Work out the finished part from the listing and answer in its coordinate system (mm). Coordinates: 2 decimals unless noted, no trailing zeros. Loops run counter-clockwise (first coordinate to the right, second up) from the corner with the lowest first, then second, coordinate; pieces in that order, holes last. Notation, with made-up numbers: (4.25, -13) - (43.25, -13) arc R32 ccw to (43.25, 16) - close; hole circle Ø10 at (76, -26.5). An arc over 180 degrees is marked (long way). Write each question's results on one line, items separated by ' | '. Start each with the question number.
1. Each of these flat-tipped pins is pushed along its axis until it touches: P1, Ø6.5, axis at x = 0, z = 127, coming from the +Y side; P2, Ø1.5, axis at x = 3, y = -9, coming from the -Z side. Where does it stop, or does it pass through?
2. Determine the mould class of faces 1 (the flat face through (-11, -10, 2)), 2 (the flat face through (0, -1.5, 2)), 3 (the cylindrical face through (-0.716, -10.152, -121.547)) for opening direction X: released by +X, released by -X, zero draft, split by the parting line, or undercut.
3. Find the intervals of material crossed by line 1 along Z through (x, y) = (0.75, -4.25); line 2 along Z through (x, y) = (-5, -12); line 3 along X through (y, z) = (-13.75, -45.5), in increasing order. Write a range as [from, to].
4. A cutting plane is placed at B-B on x = 2.75. Determine the outline of the cut face in (y, z).
5. A cutting plane is placed at A-A on y = -7. Determine the outline of the cut face in (x, z).
from build123d import *

# Parameters (mm, degrees)
F0_R     = 5.5
F1_DEPTH = 19.05
F2_DEPTH = 1.5


# Not quite as in the source:
# - a length typed as a fraction of an inch, garbled in the dataset ("3 / 203.2 mm" for 3/8 in), is restored
# - a feature names something its author has since deleted; it is built from what else it names


with BuildPart() as f1:
    # F0 (on Front) → F1 (new body)
    with BuildSketch(Plane.XZ):
        with BuildLine():
            Line((11, -127), (11, 127))
            ThreePointArc((11, 127), (7.7781745931, 134.7781745931), (0, 138))
            ThreePointArc((0, 138), (-7.7781745931, 134.7781745931), (-11, 127))
            Line((-11, 127), (-11, -127))
            ThreePointArc((-11, -127), (-7.7781745931, -134.7781745931), (0, -138))
            ThreePointArc((0, -138), (7.7781745931, -134.7781745931), (11, -127))
        make_face()
        with Locations((0, -127)):
            Circle(F0_R, mode=Mode.SUBTRACT)
        with Locations((0, -41.9999994338)):
            Circle(F0_R, mode=Mode.SUBTRACT)
        with Locations((0, 127)):
            Circle(F0_R, mode=Mode.SUBTRACT)
    extrude(amount=F1_DEPTH)

    # F0 (on Front) → F2 (cut)
    with BuildSketch(Plane.XZ):
        with BuildLine():
            Line((11, -127), (11, 127))
            ThreePointArc((11, 127), (7.7781745931, 134.7781745931), (0, 138))
            ThreePointArc((0, 138), (-7.7781745931, 134.7781745931), (-11, 127))
            Line((-11, 127), (-11, -127))
            ThreePointArc((-11, -127), (-7.7781745931, -134.7781745931), (0, -138))
            ThreePointArc((0, -138), (7.7781745931, -134.7781745931), (11, -127))
        make_face()
        with Locations((0, -127)):
            Circle(F0_R, mode=Mode.SUBTRACT)
        with Locations((0, -41.9999994338)):
            Circle(F0_R, mode=Mode.SUBTRACT)
        with Locations((0, 127)):
            Circle(F0_R, mode=Mode.SUBTRACT)
    extrude(amount=F2_DEPTH, mode=Mode.SUBTRACT)


solid = f1.part
Values:
1) P1: through | P2: z = -137.77
2) face 1: released by -X | face 2: zero draft | face 3: undercut
3) line 1: [-137.97, -132.45], [-121.55, -47.45], [-36.55, 121.55], [132.45, 137.97] | line 2: [-136.8, -129.29], [-124.71, -44.29], [-39.71, 124.71], [129.29, 136.8] | line 3: [-11, -4.24], [4.24, 11]
4) outline: (-19.05, -137.65) - (-1.5, -137.65) - (-1.5, -131.76) - (-19.05, -131.76) - close; (-19.05, -122.24) - (-1.5, -122.24) - (-1.5, -46.76) - (-19.05, -46.76) - close; (-19.05, -37.24) - (-1.5, -37.24) - (-1.5, 122.24) - (-19.05, 122.24) - close; (-19.05, 131.76) - (-1.5, 131.76) - (-1.5, 137.65) - (-19.05, 137.65) - close
5) outline: (-11, -127) arc R11 ccw to (11, -127) - (11, 127) arc R11 ccw to (-11, 127) - close; hole circle Ø11 at (0, -127); hole circle Ø11 at (0, -42); hole circle Ø11 at (0, 127)
